from build123d import *

# Parameters (mm, degrees)
F0_R     = 152.4
F1_DEPTH = 152.4
F0_R_2   = 171.45
F2_DEPTH = 6.35
F3_T     = -2.54
F4_R     = 7.62


with BuildPart() as f1:
    # F0 (on Front) → F1 (new body)
    with BuildSketch(Plane.XZ):
        Circle(F0_R)
    extrude(amount=F1_DEPTH)

    # F0 (on Front) → F2 (join)
    with BuildSketch(Plane.XZ):
        Circle(F0_R_2)
        Circle(F0_R, mode=Mode.SUBTRACT)
    extrude(amount=F2_DEPTH)

    # F3
    f3_openings = [f1.faces().sort_by_distance(p)[0] for p in [
        (0, 0, 0),
    ]]
    offset(amount=F3_T, openings=f3_openings, kind=Kind.INTERSECTION)

    # F4
    f4_edges = [f1.edges().sort_by_distance(p)[0] for p in [
        (-152.4, -152.4, 0),
        (-152.4, -6.35, 0),
        (-149.86, -149.86, 0),
    ]]
    fillet(f4_edges, radius=F4_R)


solid = f1.part
Model file for the job. Use its own axes, mm. A direction names the side the tool comes from. Give positions to 0.01 mm unless a question says otherwise; leave off trailing zeros. Order: outer loops, then holes, each group sorted by start corner. A loop starts at its lowest first (then second) coordinate and runs counter-clockwise, first axis right, second up. Notation, with made-up numbers: (-26, -0.75) - (0, -0.75) arc R29 cw to (0, 30.25) - close; hole circle Ø2 at (11, -17). An arc over 180 degrees is marked (long way). Return JSON: item names as keys, results as strings.
1) 3-axis set-ups, long thin cutter, end or side, ignore diameter. For faces 1 (the flat face through (126, 0, -113)), 2 (the cylindrical face through (77.942, -1.878, -149.852)), 3 (the cylindrical face through (-120.94, -78.46, -92.73)): which of +Z, -Z, +X, -X, +Y, -Y reach the whole face in a straight line?
Geometry says:
{"face 1": "+Z, -Z, +X, -X, +Y", "face 2": "+Y", "face 3": "-Y"}
2) Cut at C-C, the plane y = -126. Give the cut face in (x, z), plus the area to 3 significant figures.
Geometry says:
{"outline": "circle Ø304.8 at (0, 0); hole circle Ø299.72 at (0, 0)", "area": "2,410 mm²"}
3) Pull direction Z, two halves, no side cores. Call faces 4 (the cylindrical face through (-118.92, -72.06, -91.19)), 5 (the flat face through (-2, -152.4, 2)), 6 (the cylindrical face through (92.17, -3.131, 144.567)): pulls with the +Z half, pulls with the -Z half, needs draft (parallel to the pull), parting line crosses it, or undercut.
Geometry says:
{"face 4": "undercut", "face 5": "needs draft", "face 6": "parting line crosses it"}
4) Flat gauge pins, fed straight in: P1, Ø6, axis at y = -78.5, z = -130, coming from the +X side; P2, Ø3, axis at y = -86.5, z = 12, coming from the +X side; P3, Ø5, axis at x = 10, z = -15, coming from the +Y side. Where does each tip first touch, or does it go through?
Geometry says:
{"P1": "x = 84.24", "P2": "x = 152.04", "P3": "y = -149.86"}
5) Probe line 1 (Z direction, x = 0, y = -73); line 2 (Z direction, x = 0, y = -2.35); line 3 (Y direction, x = -61, z = 120). List the from-to ranges inside material, lowest first. Write a range as from..to.
Geometry says:
{"line 1": "-152.4..-149.86, 149.86..152.4", "line 2": "-171.45..-168.91, 168.91..171.45", "line 3": "-152.4..-149.86"}
6) Cut at B-B, the plane x = 0. Give the cut face in (y, z), plus the area to 3 significant figures.
Geometry says:
{"outline": "(-152.4, -144.78) arc R7.62 ccw to (-144.78, -152.4) - (-13.97, -152.4) arc R7.62 cw to (-6.35, -160.02) - (-6.35, -171.45) - (0, -171.45) - (0, -168.91) - (-3.81, -168.91) - (-3.81, -149.86) - (-142.24, -149.86) arc R7.62 cw to (-149.86, -142.24) - (-149.86, 142.24) arc R7.62 cw to (-142.24, 149.86) - (-3.81, 149.86) - (-3.81, 168.91) - (0, 168.91) - (0, 171.45) - (-6.35, 171.45) - (-6.35, 160.02) arc R7.62 cw to (-13.97, 152.4) - (-144.78, 152.4) arc R7.62 ccw to (-152.4, 144.78) - close", "area": "1,660 mm²"}
7) Cut at A-A, the plane z = 0. Give the cut face in (x, y).
Geometry says:
{"outline": "(-171.45, -6.35) - (-160.02, -6.35) arc R7.62 cw to (-152.4, -13.97) - (-152.4, -144.78) arc R7.62 ccw to (-144.78, -152.4) - (144.78, -152.4) arc R7.62 ccw to (152.4, -144.78) - (152.4, -13.97) arc R7.62 cw to (160.02, -6.35) - (171.45, -6.35) - (171.45, 0) - (168.91, 0) - (168.91, -3.81) - (149.86, -3.81) - (149.86, -142.24) arc R7.62 cw to (142.24, -149.86) - (-142.24, -149.86) arc R7.62 cw to (-149.86, -142.24) - (-149.86, -3.81) - (-168.91, -3.81) - (-168.91, 0) - (-171.45, 0) - close"}
